Part model, mm, in its own coordinate system. A direction names the side the tool comes from. Coordinates: 2 decimals unless noted, no trailing zeros. Loops run counter-clockwise (first coordinate to the right, second up) from the corner with the lowest first, then second, coordinate; pieces in that order, holes last. Notation, with made-up numbers: (59.25, 57) -> (102.25, 57) arc R31 cw to (102.25, 83) -> close; hole circle Ø7 at (17, 47.25). An arc over 180 degrees is marked (long way). One line per item, written item: value. Start each with the question number.
from build123d import *

# Parameters (mm, degrees)
SKETCH1_R           = 1.27
BOSS_EXTRUDE1_DEPTH = 1.27
BOSS_EXTRUDE2_DEPTH = 0.508


with BuildPart() as part:
    # Sketch1 → Boss-Extrude1 (new body)
    with BuildSketch(Plane.XY):
        with BuildLine():
            Line((6.924783114, -0.138801739), (-1.3615811, 11.254923221))
            ThreePointArc((-1.3615811, 11.254923221), (-3.633316734, 11.992153009), (-5.036931534, 10.059756558))
            Line((-5.036931534, 10.059756558), (-5.036931534, 2.032))
            ThreePointArc((-5.036931534, 2.032), (-4.441772513, 0.595159021), (-3.004931534, 0))
            Line((-3.004931534, 0), (0, 0))
            Line((0, 0), (0, -12.7))
            Line((0, -12.7), (7.31343268, -12.7))
            Line((7.31343268, -12.7), (7.31343268, -1.333968401))
            ThreePointArc((7.31343268, -1.333968401), (7.21382913, -0.705583202), (6.924783114, -0.138801739))
        make_face()
        with Locations((-3.004931534, 10.059756558)):
            Circle(SKETCH1_R, mode=Mode.SUBTRACT)
        with Locations((-3.004931534, 5.27395868)):
            Circle(SKETCH1_R, mode=Mode.SUBTRACT)
    extrude(amount=BOSS_EXTRUDE1_DEPTH)

    # Sketch2 → Boss-Extrude2 (add)
    with BuildSketch(Plane(origin=(0, -12.7, 0), x_dir=(-1, 0, 0), z_dir=(0, -1, 0))):
        Polygon((-7.52318228, 2.564928968), (-7.52318228, -3.846337758), (0.09681772, -3.785071032), (0.045762115, 2.564928968), align=None)
    extrude(amount=BOSS_EXTRUDE2_DEPTH)


solid = part.part
1) Slice it at D-D (z = -0.25). Give the cut face in (x, y).
2) Pull direction X, two halves, no side cores. Call faces 5 (the cylindrical face through (-3.599, 12.003, 0.626)), 6 (the cylindrical face through (-3.17, 6.533, 0.626)), 7 (the flat face through (7.313, -7, 1)): +X half, -X half, draft (parallel to the pull), parting line (faces both ways), or undercut.
3) Slice it at B-B (y = -6.25). Give the cut face in (x, z), then the cut area to 3 significant figures.
4) Probe line 1 (Z direction, x = -1.25, y = 7); line 2 (Y direction, x = 4, z = -2.25); line 3 (X direction, y = 1, z = 1). List the from-to ranges inside material, lowest first. Write a range as from..to.
5) Tool access for faces 1 (the flat face through (1, 0, 0)), 2 (the cylindrical face through (-4.457, 0.611, 0.626)), 3 (the flat face through (1, 0, 1.27)), 4 (the flat face through (0, -6, 1)): list every direction of +Z, -Z, +X, -X, +Y, -Y with a clear straight run to the whole face (end or side of a thin tool).
6) Slice it at A-A (x = -2.5). Give the cut face in (y, z), then the cut area to 3 significant figures.
7) Pin check, flat tips, straight feed: pin 1 Ø1.4 at (x, z) = (-1.5, 0.5) entering from -Y; pin 2 Ø3.5 at (x, y) = (1.5, 2.5) entering from -Z; pin 3 Ø0.6 at (y, z) = (-5, 0.5) entering from +X. Stop position of each tip, or through.
8) Slice it at C-C (x = 2.25). Give the cut face in (y, z), then the cut area to 3 significant figures.
Check sheet entries:
1. outline: (-0.06, -13.21) -> (7.52, -13.21) -> (7.52, -12.7) -> (-0.06, -12.7) -> close
2. face 5: parting line
2. face 6: undercut
2. face 7: +X half
3. outline: (0, 0) -> (7.31, 0) -> (7.31, 1.27) -> (0, 1.27) -> close
3. area: 9.29 mm^2
4. line 1: z = 0..1.27
4. line 2: y = -13.21..-12.7
4. line 3: x = -4.76..6.1
5. face 1: -Z, +X, -X, +Y
5. face 2: +Z, -Z, -X, -Y
5. face 3: +Z, +X, -X, +Y
5. face 4: +Z, -Z, -X
6. outline: (0, 0) -> (4.11, 0) -> (4.11, 1.27) -> (0, 1.27) -> close; (6.44, 0) -> (8.89, 0) -> (8.89, 1.27) -> (6.44, 1.27) -> close; (11.23, 0) -> (12.03, 0) -> (12.03, 1.27) -> (11.23, 1.27) -> close
6. area: 9.36 mm^2
7. pin 1: stops at y = 0
7. pin 2: stops at z = 0
7. pin 3: stops at x = 7.31
8. outline: (-13.21, -2.56) -> (-12.7, -2.56) -> (-12.7, 0) -> (6.29, 0) -> (6.29, 1.27) -> (-12.7, 1.27) -> (-12.7, 3.8) -> (-13.21, 3.8) -> close
8. area: 27.4 mm^2
